For this review, take the finished solid that the model builds, in its own axes (mm). Face numbers are marked on the shaded views. A direction names the side the tool comes from. Round coordinates to 2 decimals unless told otherwise and drop trailing zeros. Order: outer loops, then holes, each group sorted by start corner. A loop starts at its lowest first (then second) coordinate and runs counter-clockwise, first axis right, second up. Notation, with made-up numbers: (67, 61.5) -> (104, 61.5) arc R16 ccw to (104, 66.5) -> close; hole circle Ø4 at (43.5, 41.25). An arc over 180 degrees is marked (long way). Use a Markdown table: item, result. Add a question column.
1) Consider section A-A (y = 1). State the section outline as (x, z) points, plus the area to 3 significant figures.
2) Consider section C-C (x = 0). State the section outline as (y, z) points, plus the area to 3 significant figures.
3) Consider section D-D (y = 2.5). State the section outline as (x, z) points, plus the area to 3 significant figures.
4) Consider section B-B (z = 0). State the section outline as (x, y) points, plus the area to 3 significant figures.
5) Wall thickness on line 1 along Y through (x, z) = (2.25, -0.35); line 2 along Y through (x, z) = (1.1, 0.3); line 3 along Z through (x, y) = (-0.5, 4.25): over which ranges is each line inside the solid? List them lowest first. Write a range as [from, to].
6) Clearance check with flat-ended pins moving along their axes: P1, Ø0.8, axis at x = -1, y = 0.5, coming from the +Z side; P2, Ø0.8, axis at x = -1.5, y = 1, coming from the -Z side; P3, Ø1.2, axis at y = 1, z = 1, coming from the +X side. State where each tip first meets the part, or that it passes through.
7) Machinability: for the marked faces 1 and 2, which of the approach directions +Z, -Z, +X, -X, +Y, -Y give a long, thin tool a straight path to every point of the face, cutting with its end or side? Answer none if there is none.
8) Draft analysis for pull direction Z (two halves, no side actions). For the marked faces 3, 4 and 5, state which applies: pulls with the +Z half, pulls with the -Z half, needs draft (parallel to the pull), parting line crosses it, or undercut.
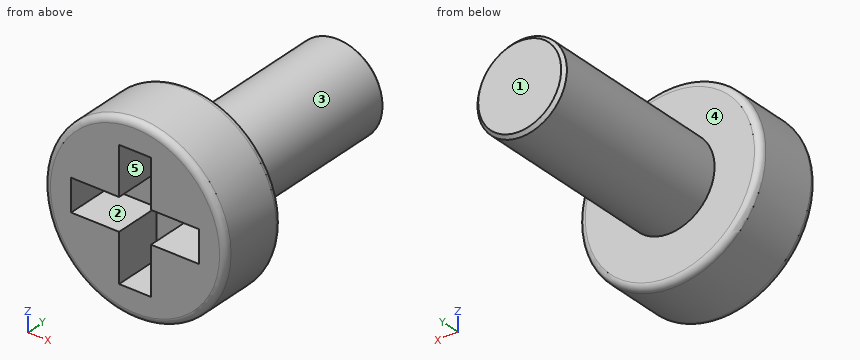
```python
from build123d import *

# Parameters (mm, degrees)
SKETCH_1_R          = 2.85
EXTRUDE_1_DEPTH     = 2.2
SKETCH_2_R          = 1.4
EXTRUDE_2_DEPTH     = 6
CHAMFER_1_SIZE      = 0.1
FILLET_1_R          = 0.2
CUT_EXTRUDE_1_DEPTH = 1.5


with BuildPart() as part:
    # Эскиз1 → Бобышка-Вытянуть1 (new body)
    with BuildSketch(Plane(origin=(0, 0, 0), x_dir=(1, 0, 0), z_dir=(0, 1, 0))):
        Circle(SKETCH_1_R)
    extrude(amount=EXTRUDE_1_DEPTH)

    # Эскиз2 → Бобышка-Вытянуть2 (add)
    with BuildSketch(Plane(origin=(0, 2.2, 0), x_dir=(1, 0, 0), z_dir=(0, 1, 0))):
        Circle(SKETCH_2_R)
    extrude(amount=EXTRUDE_2_DEPTH)

    # Фаска1
    chamfer_1_edges = [part.edges().sort_by_distance(p)[0] for p in [
        (-1.4, 8.2, 0),
    ]]
    chamfer(chamfer_1_edges, length=CHAMFER_1_SIZE)

    # Скругление1
    fillet_1_edges = [part.edges().sort_by_distance(p)[0] for p in [
        (-2.85, 0, 0),
        (-2.85, 2.2, 0),
    ]]
    fillet(fillet_1_edges, radius=FILLET_1_R)

    # Эскиз3 → Вырез-Вытянуть1 (cut)
    with BuildSketch(Plane.XZ):
        Polygon((-0.5, 0.5), (-0.5, 2), (0.5, 2), (0.5, 0.5), (2, 0.5), (2, -0.5), (0.5, -0.5), (0.5, -2), (-0.5, -2), (-0.5, -0.5), (-2, -0.5), (-2, 0.5), align=None)
    extrude(amount=-CUT_EXTRUDE_1_DEPTH, mode=Mode.SUBTRACT)


solid = part.part
```
Results list:
| question | item | result |
|---|---|---|
| 1 | outline | circle Ø5.7 at (0, 0); hole (-2, -0.5) -> (-0.5, -0.5) -> (-0.5, -2) -> (0.5, -2) -> (0.5, -0.5) -> (2, -0.5) -> (2, 0.5) -> (0.5, 0.5) -> (0.5, 2) -> (-0.5, 2) -> (-0.5, 0.5) -> (-2, 0.5) -> close |
| 1 | area | 18.5 mm2 |
| 2 | outline | (0, -2.65) arc R0.2 ccw to (0.2, -2.85) -> (2, -2.85) arc R0.2 ccw to (2.2, -2.65) -> (2.2, -1.4) -> (8.1, -1.4) -> (8.2, -1.3) -> (8.2, 1.3) -> (8.1, 1.4) -> (2.2, 1.4) -> (2.2, 2.65) arc R0.2 ccw to (2, 2.85) -> (0.2, 2.85) arc R0.2 ccw to (0, 2.65) -> (0, 2) -> (1.5, 2) -> (1.5, -2) -> (0, -2) -> close |
| 2 | area | 23.3 mm2 |
| 3 | outline | circle Ø2.8 at (0, 0) |
| 3 | area | 6.16 mm2 |
| 4 | outline | (-2.85, 0.2) arc R0.2 ccw to (-2.65, 0) -> (-2, 0) -> (-2, 1.5) -> (2, 1.5) -> (2, 0) -> (2.65, 0) arc R0.2 ccw to (2.85, 0.2) -> (2.85, 2) arc R0.2 ccw to (2.65, 2.2) -> (1.4, 2.2) -> (1.4, 8.1) -> (1.3, 8.2) -> (-1.3, 8.2) -> (-1.4, 8.1) -> (-1.4, 2.2) -> (-2.65, 2.2) arc R0.2 ccw to (-2.85, 2) -> close |
| 4 | area | 23.3 mm2 |
| 5 | line 1 | [0, 2.2] |
| 5 | line 2 | [1.5, 8.2] |
| 5 | line 3 | [-1.31, 1.31] |
| 6 | P1 | z = 2.79 |
| 6 | P2 | z = -2.63 |
| 6 | P3 | x = 2.82 |
| 7 | face 1 | +Z, -Z, +X, -X, +Y |
| 7 | face 2 | -Y |
| 8 | face 3 | parting line crosses it |
| 8 | face 4 | needs draft |
| 8 | face 5 | undercut |
